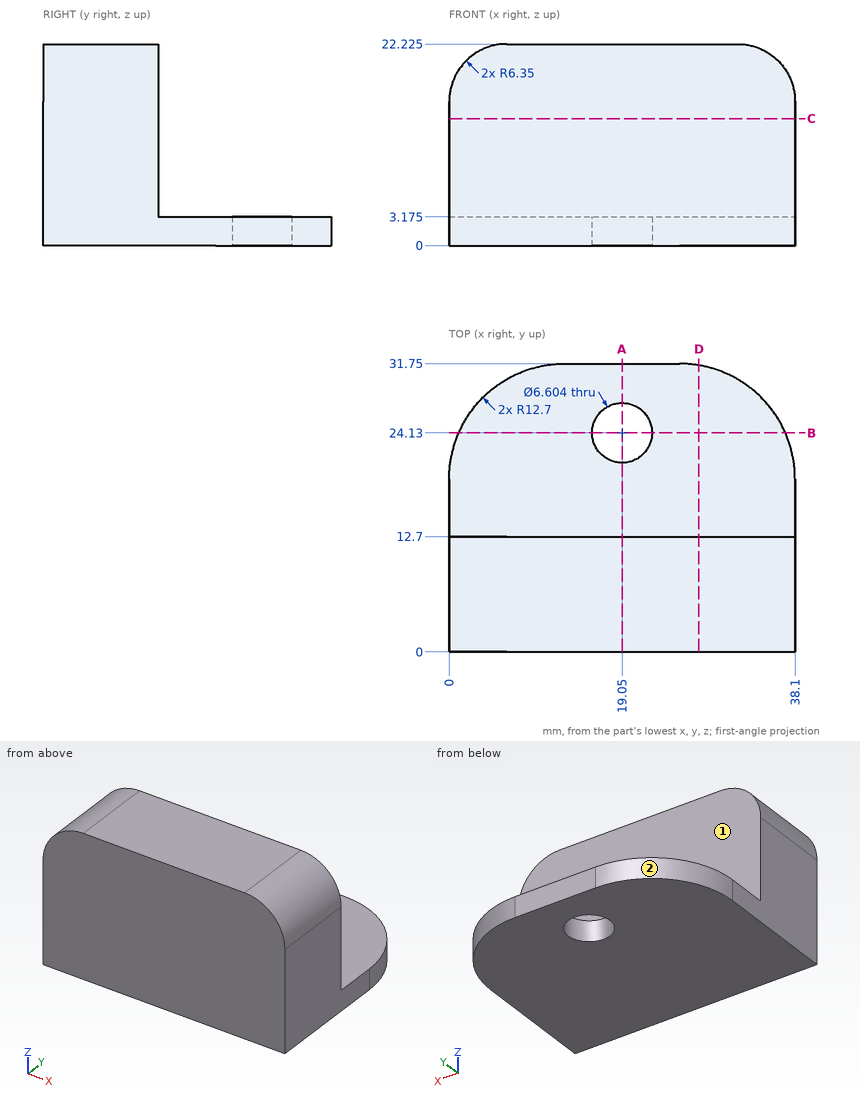
Design review of the part shown in the three views and the two pictorial views. Dimensions are in mm from the part's minimum x, y and z. A direction names the side the tool comes from. Give positions to 0.01 mm unless a question says otherwise; leave off trailing zeros. Write each loop counter-clockwise with the first axis right and the second up, starting at its lowest first coordinate (ties: lowest second). Pieces come first, ordered by that corner, then holes. Notation, with made-up numbers: M 88.25,-35 L 125.25,-35 A19 cw 125.25,-31 Z; hole C 36,21 d1. An arc over 180 degrees is marked long. Answer as CSV lines item,"result".
1. Consider section C-C, the plane z = 14. Write out the cut boundary in (x, y).
Findings:
outline,"M 0,0 L 38.1,0 L 38.1,12.7 L 0,12.7 Z"
2. For pin 1 (10.5 mm diameter, centred on x = 19.05, y = 24.13, fed in from -Z); pin 2 (8 mm diameter, centred on x = 12.5, z = 10, fed in from +Y); pin 3 (3 mm diameter, centred on x = 7.5, y = 15, fed in from +Z) (3 decimals), all flat-tipped, find the tip position at first contact; note any pin that passes through.
Findings:
pin 1,"stops at z = 0"
pin 2,"stops at y = 12.7"
pin 3,"stops at z = 3.175"
3. Consider section A-A, the plane x = 19.05. Write out the cut boundary in (y, z) (3 decimals), then the cut area to 3 significant figures.
Findings:
outline,"M 0,0 L 20.828,0 L 20.828,3.175 L 12.7,3.175 L 12.7,22.225 L 0,22.225 Z; M 27.432,0 L 31.75,0 L 31.75,3.175 L 27.432,3.175 Z"
area,"322 mm2"
4. For the marked faces 1 and 2, list the 3-axis set-ups (+Z, -Z, +X, -X, +Y, -Y) from which the entire face can be reached by the end or side of a thin tool; tool diameter is ignored.
Findings:
face 1,"+Z, +X, -X, +Y"
face 2,"+Z, -Z, -X, +Y"
5. Consider section D-D, the plane x = 27.5. Write out the cut boundary in (y, z) (3 decimals), then the cut area to 3 significant figures.
Findings:
outline,"M 0,0 L 31.575,0 L 31.575,3.175 L 12.7,3.175 L 12.7,22.225 L 0,22.225 Z"
area,"342 mm2"
6. Consider section B-B, the plane y = 24.13. Write out the cut boundary in (x, z) (3 decimals).
Findings:
outline,"M 1.06,0 L 15.748,0 L 15.748,3.175 L 1.06,3.175 Z; M 22.352,0 L 37.04,0 L 37.04,3.175 L 22.352,3.175 Z"
7. Wall thickness on line 1 (Y direction, x = 19.05, z = 1); line 2 (Y direction, x = 6, z = 13); line 3 (Z direction, x = 27, y = 22.5) (3 decimals): over which ranges is each line inside the solid? List them lowest first.
Findings:
line 1,"y = 0 to 20.83, 27.43 to 31.75"
line 2,"y = 0 to 12.7"
line 3,"z = 0 to 3.175"
